Could you check a few things on this model? Use its own coordinates, in mm. Give positions to 0.01 mm unless a question says otherwise; leave off trailing zeros. Order: outer loops, then holes, each group sorted by start corner. A loop starts at its lowest first (then second) coordinate and runs counter-clockwise, first axis right, second up. Notation, with made-up numbers: (64, -38) -> (95, -38) arc R20 ccw to (95, -18) -> close; hole circle Ø5 at (-7.5, 17.5). An arc over 180 degrees is marked (long way). Answer as CSV lines item,"result". Start each with the question number.
(1) I need wall thicknesses on L1, parallel to X at y = 272, z = 639.5; L2, parallel to X at y = -67.5, z = 75.5. Which ranges of each line are inside material? Lowest first, please.
(2) Will these pins go through, and if not, where does the flat tip stop? pin 1 Ø22.5 at (x, z) = (319, 691) entering from +Y; pin 2 Ø7.5 at (y, z) = (-67.5, 818.5) entering from +X; pin 3 Ø7.5 at (x, y) = (288.5, -100) entering from -Z; pin 4 Ø10 at (y, z) = (22, 539.5) entering from +X.
(3) I want a section at A-A (y = 82.5). Please give me the cut outline in (x, z).
(4) I want a section at B-B (z = 484.5). Please give me the cut outline in (x, y), plus the area to 3 significant figures.
```python
from build123d import *

# Parameters (mm, degrees)
F0_W        = 600
F0_H        = 600
F1_DEPTH    = 800
F2_W        = 600
F2_H        = 80
F3_DEPTH    = 25
F5_DEPTH    = 50
F6_T1_DEPTH = 120
F6_T4_ANGLE = 180
F6_T6_ANGLE = 180
F7_W        = 40
F7_H        = 110
F8_DEPTH    = 25
F9_R        = 4.99999
F10_W       = 630
F10_H       = 600
F11_DEPTH   = 25


# Not quite as in the source:
# - a fillet or chamfer that OpenCascade refuses, or shapes differently, is made with other operations: its cross-section is extruded or revolved along the edge and cut away or added
# - a fillet or chamfer is up to 0.001 mm smaller than in the source, because OpenCascade refuses the exact size


with BuildPart() as f1:
    # F0 (on Top) → F1 (new body)
    with BuildSketch(Plane.XY):
        Rectangle(F0_W, F0_H)
    extrude(amount=F1_DEPTH)

    # F2 (on face) → F3 (cut)
    with BuildSketch(Plane.YZ.offset(300)):
        with Locations((0, 40)):
            Rectangle(F2_W, F2_H)
    extrude(amount=-F3_DEPTH, mode=Mode.SUBTRACT)

    # F4 (on face) → F5 (join)
    with BuildSketch(Plane.YZ.offset(300)):
        with BuildLine():
            ThreePointArc((-248.5795542598, 750), (-252.1150881657, 748.5355339059), (-253.5795542598, 745))
            Line((-253.5795542598, 745), (-253.5795542598, 625))
            ThreePointArc((-253.5795542598, 625), (-252.1150881657, 621.4644660941), (-248.5795542598, 620))
            ThreePointArc((-248.5795542598, 620), (-245.0440203538, 621.4644660941), (-243.5795542598, 625))
            Line((-243.5795542598, 625), (-243.5795542598, 745))
            ThreePointArc((-243.5795542598, 745), (-245.0440203538, 748.5355339059), (-248.5795542598, 750))
        make_face()
    extrude(amount=F5_DEPTH)

    # F6: fillet of radius 5 on 4 edges, made by hand

    # F6_s2 → F6_t1 (cut)
    with BuildSketch(Plane.XY.offset(625)):
        with BuildLine():
            ThreePointArc((345, -253.5795542598), (348.5355339059, -252.1150881657), (350, -248.5795542598))
            Line((350, -248.5795542598), (350, -253.5795542598))
            Line((350, -253.5795542598), (345, -253.5795542598))
        make_face()
        with BuildLine():
            ThreePointArc((345, -243.5795542598), (348.5355339059, -245.0440203538), (350, -248.5795542598))
            Line((350, -248.5795542598), (350, -243.5795542598))
            Line((350, -243.5795542598), (345, -243.5795542598))
        make_face()
    extrude(amount=F6_T1_DEPTH, mode=Mode.SUBTRACT)

    # F6_s3 → F6_t4 (revolve, cut)
    with BuildSketch(Plane.XY.offset(745)):
        with BuildLine():
            ThreePointArc((345, -253.5795542598), (348.5355339059, -252.1150881657), (350, -248.5795542598))
            Line((350, -248.5795542598), (350, -253.5795542598))
            Line((350, -253.5795542598), (345, -253.5795542598))
        make_face()
    revolve(axis=Axis((350, -248.5795542598, 745), (-1, 0, 0)), revolution_arc=F6_T4_ANGLE, mode=Mode.SUBTRACT)

    # F6_s5 → F6_t6 (revolve, cut)
    with BuildSketch(Plane.XY.offset(625)):
        with BuildLine():
            ThreePointArc((345, -243.5795542598), (348.5355339059, -245.0440203538), (350, -248.5795542598))
            Line((350, -248.5795542598), (350, -243.5795542598))
            Line((350, -243.5795542598), (345, -243.5795542598))
        make_face()
    revolve(axis=Axis((350, -248.5795542598, 625), (-1, 0, 0)), revolution_arc=F6_T6_ANGLE, mode=Mode.SUBTRACT)

    # F7 (on face) → F8 (cut)
    with BuildSketch(Plane(origin=(0, -243.5795542598, 0), x_dir=(-1, 0, 0), z_dir=(0, 1, 0))):
        with Locations((-320, 685)):
            Rectangle(F7_W, F7_H)
    extrude(amount=-F8_DEPTH, mode=Mode.SUBTRACT)

    # F9 (radius 5 in the source; OpenCascade refuses exactly that, so slightly less here)
    f9_edges = [f1.edges().sort_by_distance(p)[0] for p in [
        (320, -243.579554, 740),
        (340, -243.579554, 685),
        (320, -243.579554, 630),
        (320, -253.579554, 740),
        (340, -253.579554, 685),
        (320, -253.579554, 630),
    ]]
    fillet(f9_edges, radius=F9_R)

    # F10 (on face) → F11 (join)
    with BuildSketch(Plane.XY.offset(800)):
        with Locations((15, 0)):
            Rectangle(F10_W, F10_H)
    extrude(amount=F11_DEPTH)


solid = f1.part
```
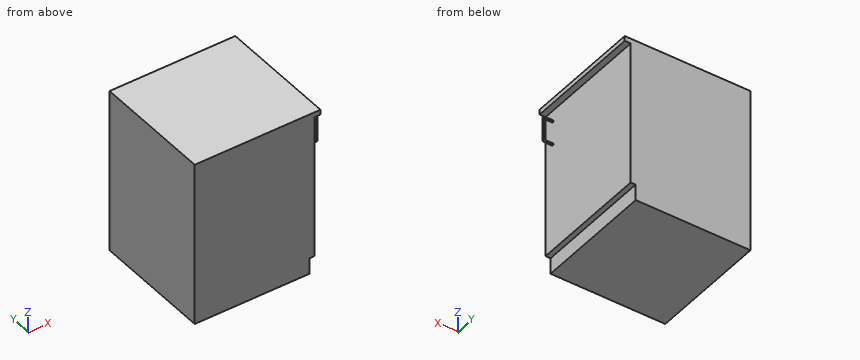
Final values:
1,L1,"-300 to 300"
1,L2,"-300 to 275"
2,pin 1,"through"
2,pin 2,"x = 330"
2,pin 3,"z = 80"
2,pin 4,"x = 300"
3,outline,"(-300, 0) -> (275, 0) -> (275, 80) -> (300, 80) -> (300, 800) -> (330, 800) -> (330, 825) -> (-300, 825) -> close"
4,outline,"(-300, -300) -> (300, -300) -> (300, 300) -> (-300, 300) -> close"
4,area,"360,000 mm²"
